from build123d import *

# Parameters (mm, degrees)
TD_SKETCH_R                  = 1.58623
TL_FEATURE_DEPTH             = 63.5
TDF_SKETCH_W                 = 3.19246
TDF_SKETCH_H                 = 3.19246
TDF_FEATURE_DEPTH            = 64.53961167
ISA_FEATURE_DEPTH            = 64.53961167
ISA_FEATURE_DEPTH_BACK       = 64.53961167
STD_SHANK_FEATURE_DEPTH      = 64.53961167
STD_SHANK_FEATURE_DEPTH_BACK = 64.53961167


with BuildPart() as part:
    # TD_sketch → TL_feature (new body)
    with BuildSketch(Plane(origin=(0, 0, 0), x_dir=(1, 0, 0), z_dir=(0, 1, 0))):
        with Locations(Location((0, 0, 0), (0, 0, 270))):
            Circle(TD_SKETCH_R)
    extrude(amount=TL_FEATURE_DEPTH)

    # TDF_sketch → TDF_feature (cut, through all)
    with BuildSketch(Plane(origin=(0, 0, 0), x_dir=(1, 0, 0), z_dir=(0, 1, 0))):
        with Locations((-2.804, 0)):
            Rectangle(TDF_SKETCH_W, TDF_SKETCH_H)
    extrude(amount=TDF_FEATURE_DEPTH, mode=Mode.SUBTRACT)

    # ISA_sketch → ISA_feature (cut, two sides: drawn at the far end of the back side and taken through both)
    with BuildSketch(Plane(origin=(0, 0, 0), x_dir=(0, 0, -1), z_dir=(1, 0, 0)).offset(-ISA_FEATURE_DEPTH_BACK)):
        Polygon((-54.007028628, 201.05930583), (-17.148123719, 63.5), (-0.13335, 0), (0.13335, 0), (17.148123719, 63.5), (54.007028628, 201.05930583), (54.007028628, -83.764439609), (-54.007028628, -83.764439609), align=None)
    extrude(amount=ISA_FEATURE_DEPTH + ISA_FEATURE_DEPTH_BACK, mode=Mode.SUBTRACT)

    # STD_shank_sketch → STD_shank_feature (cut, two sides: drawn at the far end of the back side and taken through both)
    with BuildSketch(Plane.XY.offset(-STD_SHANK_FEATURE_DEPTH_BACK)):
        Polygon((-17.472069957, 200.795385926), (-5.460280134, 63.5), (0.09525, 0), (0.46355, 0), (6.019080134, 63.5), (18.030869957, 200.795385926), (18.030869957, -74.844278065), (-17.472069957, -74.844278065), align=None)
    extrude(amount=STD_SHANK_FEATURE_DEPTH + STD_SHANK_FEATURE_DEPTH_BACK, mode=Mode.SUBTRACT)


solid = part.part
The listing builds one solid part. Answer for the finished solid, in the listing's coordinates (mm). Coordinates: 2 decimals unless noted, no trailing zeros. Loops run counter-clockwise (first coordinate to the right, second up) from the corner with the lowest first, then second, coordinate; pieces in that order, holes last. Notation, with made-up numbers: M 65,89 L 117,89 A31 ccw 117,124 Z; hole C 84.5,-8.5 d7. An arc over 180 degrees is marked long. Answer in a Markdown table with one row per item.
1) Find the intervals of material crossed by probe 1 along Z at (x, y) = (0.1, 40); probe 2 along X at (y, z) = (32, 0.1); probe 3 along X at (y, z) = (23.5, 0.35), in increasing order.
Answers below:
| item | result |
|---|---|
| probe 1 | -1.58 to 1.58 |
| probe 2 | -1.21 to 1.58 |
| probe 3 | -1.21 to 1.55 |
2) Given pin 1 (1.5 mm diameter, centred on y = 41, z = 1, fed in from +X), flat-ended and moving along its own axis, determine where the tip first touches the part or whether it passes through.
Answers below:
| item | result |
|---|---|
| pin 1 | x = 1.57 |
3) Find section A-A (y = 43). Determine the outline of the cut face in (x, z), then the cut area to 3 significant figures.
Answers below:
| item | result |
|---|---|
| outline | M -1.21,-1.03 A1.59 ccw long -1.21,1.03 Z |
| area | 7.37 mm^2 |
